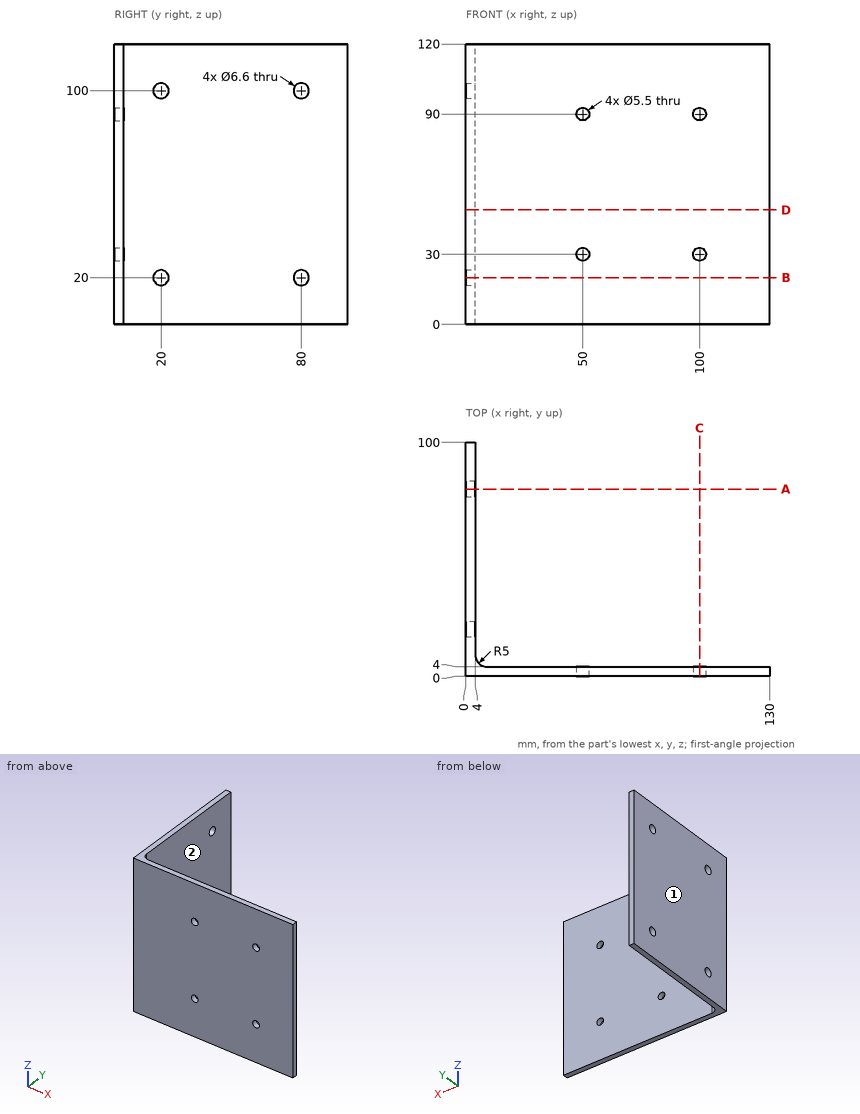
Drawing for the job (mm, zero at the part's lowest x, y, z). A direction names the side the tool comes from. Round coordinates to 2 decimals unless told otherwise and drop trailing zeros. Write each loop counter-clockwise with the first axis right and the second up, starting at its lowest first coordinate (ties: lowest second). Pieces come first, ordered by that corner, then holes. Notation, with made-up numbers: M 57.5,-27 L 78.5,-27 A23 ccw 78.5,-6 Z; hole C 9,48 d7. An arc over 180 degrees is marked long. One line per question, with ' | ' between items.
1. Probe L1, parallel to Z at x = 0.9, y = 20; L2, parallel to Z at x = 50, y = 1.55; L3, parallel to Y at x = 19, z = 11. List the from-to ranges inside material, lowest first. Write a range as from..to.
Working result:
L1: 0..16.7, 23.3..96.7, 103.3..120 | L2: 0..27.25, 32.75..87.25, 92.75..120 | L3: 0..4
2. Cut at B-B on z = 20. Write the cut outline in (x, y).
Working result:
outline: M 0,0 L 130,0 L 130,4 L 9,4 A5 cw 4,9 L 4,16.7 L 0,16.7 Z; M 0,23.3 L 4,23.3 L 4,76.7 L 0,76.7 Z; M 0,83.3 L 4,83.3 L 4,100 L 0,100 Z
3. Cut at A-A on y = 80. Write the cut outline in (x, z).
Working result:
outline: M 0,0 L 4,0 L 4,16.7 L 0,16.7 Z; M 0,23.3 L 4,23.3 L 4,96.7 L 0,96.7 Z; M 0,103.3 L 4,103.3 L 4,120 L 0,120 Z
4. Which spindle directions (+Z, -Z, +X, -X, +Y, -Y) get a long thin tool onto all of the face, cutting with end or side? Do the marked faces 1 and 2. Say none if no direction does.
Working result:
face 1: +Z, -Z, -X, +Y, -Y | face 2: +Z, -Z, +X, +Y
5. Pin check, flat tips, straight feed: pin 1 Ø1.5 at (y, z) = (59, 38) entering from +X; pin 2 Ø7 at (x, z) = (100, 30) entering from +Y. Stop position of each tip, or through.
Working result:
pin 1: x = 4 | pin 2: y = 4
6. Cut at D-D on z = 49. Write the cut outline in (x, y), and give its area (3 significant figures).
Working result:
outline: M 0,0 L 130,0 L 130,4 L 9,4 A5 cw 4,9 L 4,100 L 0,100 Z | area: 909 mm2
7. Cut at C-C on x = 100. Write the cut outline in (y, z), and give its area (3 significant figures).
Working result:
outline: M 0,0 L 4,0 L 4,27.25 L 0,27.25 Z; M 0,32.75 L 4,32.75 L 4,87.25 L 0,87.25 Z; M 0,92.75 L 4,92.75 L 4,120 L 0,120 Z | area: 436 mm2
